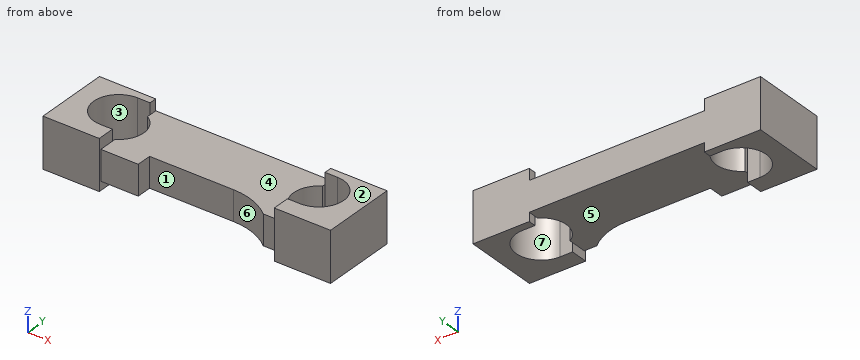
from build123d import *

# Parameters (mm, degrees)
SKETCH1_W           = 292.1
SKETCH1_H           = 50.8
BOSS_EXTRUDE1_DEPTH = 76.2
SKETCH2_W           = 177.8
SKETCH2_H           = 11.43
SKETCH2_H_2         = 8.89
CUT_EXTRUDE1_DEPTH  = 307.120058147
SKETCH3_W           = 177.8
SKETCH3_H           = 30.48
CUT_EXTRUDE2_DEPTH  = 2.032
SKETCH4_W           = 139.7
SKETCH4_H           = 30.48
CUT_EXTRUDE3_DEPTH  = 15.24
SKETCH5_W           = 12.7
SKETCH5_H           = 30.48
BOSS_EXTRUDE2_DEPTH = 15.24
FILLET1_R           = 64.77
CUT_EXTRUDE4_DEPTH  = 307.120058147
CUT_EXTRUDE5_DEPTH  = 307.120058147


with BuildPart() as part:
    # Sketch1 → Boss-Extrude1 (new body)
    with BuildSketch(Plane(origin=(0, 0, 0), x_dir=(1, 0, 0), z_dir=(0, 1, 0))):
        with Locations((146.05, 25.4)):
            Rectangle(SKETCH1_W, SKETCH1_H)
    extrude(amount=BOSS_EXTRUDE1_DEPTH)

    # Sketch2 → Cut-Extrude1 (cut, through all)
    with BuildSketch(Plane.XZ):
        with Locations((146.05, -5.715)):
            Rectangle(SKETCH2_W, SKETCH2_H)
        with Locations((146.05, -46.355)):
            Rectangle(SKETCH2_W, SKETCH2_H_2)
    extrude(amount=-CUT_EXTRUDE1_DEPTH, mode=Mode.SUBTRACT)

    # Sketch3 → Cut-Extrude2 (cut)
    with BuildSketch(Plane.XZ):
        with Locations((146.05, -26.67)):
            Rectangle(SKETCH3_W, SKETCH3_H)
    extrude(amount=-CUT_EXTRUDE2_DEPTH, mode=Mode.SUBTRACT)

    # Sketch4 → Cut-Extrude3 (cut)
    with BuildSketch(Plane.XZ.offset(-2.032)):
        with Locations((165.1, -26.67)):
            Rectangle(SKETCH4_W, SKETCH4_H)
    extrude(amount=-CUT_EXTRUDE3_DEPTH, mode=Mode.SUBTRACT)

    # Sketch5 → Boss-Extrude2 (add)
    with BuildSketch(Plane.XZ.offset(-17.272)):
        with Locations((228.6, -26.67)):
            Rectangle(SKETCH5_W, SKETCH5_H)
    extrude(amount=BOSS_EXTRUDE2_DEPTH)

    # Fillet1
    # the kernel refuses this fillet: 64.77 mm, written as the material it adds along each edge
    with BuildSketch(Plane(origin=(222.25, 17.272, -41.91), x_dir=(0, -1, 0), z_dir=(0, 0, 1))) as fillet1_piece_1:
        with BuildLine():
            CenterArc((64.77, -41.736458882), FILLET1_R, 139.880833102, 40.119166898)
            Line((0, -41.736458882), (-1.2954, -41.736458882))
            Line((-1.2954, -41.736458882), (-1.2954, 0))
            Line((-1.2954, 0), (0, 1.2954))
            ThreePointArc((0, 1.2954), (7.62, 1.2954), (14.2494, 0.834729178))
            Line((14.2494, 0.834729178), (15.24, 0))
        make_face()
    extrude(amount=30.48)

    # Sketch6 → Cut-Extrude4 (cut, through all)
    with BuildSketch(Plane.XY):
        with BuildLine():
            Line((44.45, 17.78), (57.15, 17.78))
            Line((57.15, 17.78), (57.15, 21.182954744))
            ThreePointArc((57.15, 21.182954744), (69.85, 43.18), (57.15, 65.177045256))
            Line((57.15, 65.177045256), (57.15, 68.58))
            Line((57.15, 68.58), (44.45, 68.58))
            ThreePointArc((44.45, 68.58), (19.05, 43.18), (44.45, 17.78))
        make_face()
    extrude(amount=-CUT_EXTRUDE4_DEPTH, mode=Mode.SUBTRACT)

    # Sketch7 → Cut-Extrude5 (cut, through all)
    with BuildSketch(Plane.XY):
        with BuildLine():
            Line((247.65, 17.78), (234.95, 17.78))
            Line((234.95, 17.78), (234.95, 21.182954744))
            ThreePointArc((234.95, 21.182954744), (222.25, 43.18), (234.95, 65.177045256))
            Line((234.95, 65.177045256), (234.95, 68.58))
            Line((234.95, 68.58), (247.65, 68.58))
            ThreePointArc((247.65, 68.58), (273.05, 43.18), (247.65, 17.78))
        make_face()
    extrude(amount=-CUT_EXTRUDE5_DEPTH, mode=Mode.SUBTRACT)


solid = part.part
Can you work these out from the model? Positions are in its coordinate system, mm. Face numbers are marked on the shaded views. A direction names the side the tool comes from. Give positions to 0.01 mm unless a question says otherwise; leave off trailing zeros. Loops run counter-clockwise (first coordinate to the right, second up) from the corner with the lowest first, then second, coordinate; pieces in that order, holes last. Notation, with made-up numbers: (39.25, -6.5) - (47.25, -6.5) arc R17 cw to (47.25, 11.5) - close; hole circle Ø9 at (-27, -28). An arc over 180 degrees is marked (long way). Return JSON: item names as keys, results as strings.
1. For the marked faces 4, 5, 6 and 7, which set-ups out of +Z, -Z, +X, -X, +Y, -Y let a thin tool reach every point of the face, with its end or its side?
Output values:
{"face 4": "+Z, +Y, -Y", "face 5": "-Z, +Y, -Y", "face 6": "+Z, -Z, -Y", "face 7": "+Z, -Z"}
2. I want a section at B-B on z = -2.5. Please give me the cut outline in (x, y).
Output values:
{"outline": "(0, 0) - (57.15, 0) - (57.15, 17.78) - (44.45, 17.78) arc R25.4 cw to (44.45, 68.58) - (57.15, 68.58) - (57.15, 76.2) - (0, 76.2) - close; (234.95, 0) - (292.1, 0) - (292.1, 76.2) - (234.95, 76.2) - (234.95, 68.58) - (247.65, 68.58) arc R25.4 cw to (247.65, 17.78) - (234.95, 17.78) - close"}
3. I want a section at C-C on z = -32. Please give me the cut outline in (x, y), and give its area (3 significant figures).
Output values:
{"outline": "(0, 0) - (57.15, 0) - (57.15, 2.03) - (95.25, 2.03) - (95.25, 17.27) - (180.51, 17.27) arc R64.77 cw to (222.25, 2.03) - (234.95, 2.03) - (234.95, 0) - (292.1, 0) - (292.1, 76.2) - (0, 76.2) - close; hole (44.45, 17.78) - (57.15, 17.78) - (57.15, 21.18) arc R25.4 ccw to (57.15, 65.18) - (57.15, 68.58) - (44.45, 68.58) arc R25.4 ccw to start; hole (234.95, 17.78) - (247.65, 17.78) arc R25.4 ccw to (247.65, 68.58) - (234.95, 68.58) - (234.95, 65.18) arc R25.4 ccw to (234.95, 21.18) - close", "area": "16,100 mm²"}
4. I want a section at A-A on y = 43.18. Please give me the cut outline in (x, z).
Output values:
{"outline": "(0, -50.8) - (19.05, -50.8) - (19.05, 0) - (0, 0) - close; (69.85, -41.91) - (222.25, -41.91) - (222.25, -11.43) - (69.85, -11.43) - close; (273.05, -50.8) - (292.1, -50.8) - (292.1, 0) - (273.05, 0) - close"}
5. I want a section at D-D on x = 225.5. Please give me the cut outline in (y, z).
Output values:
{"outline": "(2.03, -41.91) - (30.75, -41.91) - (30.75, -11.43) - (2.03, -11.43) - close; (55.61, -41.91) - (76.2, -41.91) - (76.2, -11.43) - (55.61, -11.43) - close"}
6. If I drill on line 1 (X direction, y = 42.5, z = -31.5); line 2 (Y direction, x = 49, z = -39.5); line 3 (X direction, y = 31.5, z = -38.5), over which ranges is the centre line in solid material (lowest first)?
Output values:
{"line 1": "x = 0 to 19.06, 69.84 to 222.26, 273.04 to 292.1", "line 2": "y = 0 to 17.78, 68.58 to 76.2", "line 3": "x = 0 to 21.89, 67.01 to 225.09, 270.21 to 292.1"}
7. I'm going to push flat-ended pins straight in: pin 1 Ø6 at (x, y) = (210, 49.5) entering from +Z; pin 2 Ø4 at (x, y) = (158.5, 38) entering from -Z; pin 3 Ø2 at (x, z) = (156, -19) entering from -Y. Where does each tip first touch, or does it pass through?
Output values:
{"pin 1": "stops at z = -11.43", "pin 2": "stops at z = -41.91", "pin 3": "stops at y = 17.27"}
8. We'd pull the mould along Y, two halves only. Please class the marked faces 1, 2 and 3: +Y half, -Y half, draft (parallel to the pull), parting line (faces both ways), or undercut.
Output values:
{"face 1": "-Y half", "face 2": "draft", "face 3": "undercut"}
